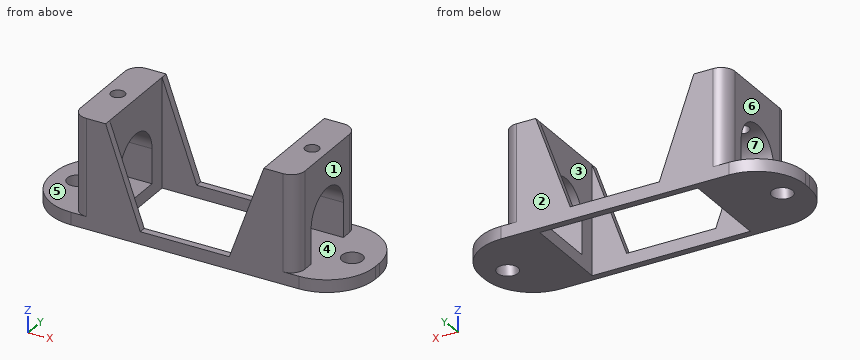
from build123d import *

# Parameters (mm, degrees)
F0_W      = 47
F0_H      = 15
F1_DEPTH  = 1.8
F3_DEPTH  = 14
F4_W      = 22.9
F4_H      = 13
F5_DEPTH  = 15.801
F6_R      = 1
F7_DEPTH  = 7
F8_R      = 1.5
F9_R      = 1.5
F10_DEPTH = 1.801
F12_DEPTH = 39.751
F13_R     = 7
F15_DEPTH = 1.001
F16_DEPTH = 14.001
F17_R     = 2


with BuildPart() as f1:
    # F0 (on Top) → F1 (new body)
    with BuildSketch(Plane.XY):
        with Locations((23.5, 7.5)):
            Rectangle(F0_W, F0_H)
    extrude(amount=F1_DEPTH)

    # F2 (on face) → F3 (join)
    with BuildSketch(Plane.XY.offset(1.8)):
        Polygon((39.75, 15), (23.5, 15), (7.25, 15), (7.25, 0), (23.5, 0), (39.75, 0), align=None)
    extrude(amount=F3_DEPTH)

    # F4 (on face) → F5 (cut, through all)
    with BuildSketch(Plane.XY.offset(15.8)):
        with Locations((23.5, 7.5)):
            Rectangle(F4_W, F4_H)
    extrude(amount=-F5_DEPTH, mode=Mode.SUBTRACT)

    # F6 (on face) → F7 (cut)
    with BuildSketch(Plane.XY.offset(15.8)):
        with Locations((9.45, 7.5)):
            Circle(F6_R)
        with Locations((37.55, 7.5)):
            Circle(F6_R)
    extrude(amount=-F7_DEPTH, mode=Mode.SUBTRACT)

    # F8 (on face) + F9 (on face) → F10 (cut, through all)
    with BuildSketch(Plane.XY.offset(1.8)):
        with Locations((3.625, 7.5)):
            Circle(F8_R)
    with BuildSketch(Plane.XY.offset(1.8)):
        with Locations((43.375, 7.5)):
            Circle(F9_R)
    extrude(amount=-F10_DEPTH, mode=Mode.SUBTRACT)

    # F11 (on face) → F12 (cut, through all)
    with BuildSketch(Plane(origin=(7.25, 0, 0), x_dir=(0, -1, 0), z_dir=(-1, 0, 0))):
        with BuildLine():
            Line((-11.5, 1.8), (-3.5, 1.8))
            Line((-3.5, 1.8), (-3.5, 6.8))
            ThreePointArc((-3.5, 6.8), (-7.5, 10.8), (-11.5, 6.8))
            Line((-11.5, 6.8), (-11.5, 1.8))
        make_face()
    extrude(amount=-F12_DEPTH, mode=Mode.SUBTRACT)

    # F13
    f13_edges = [f1.edges().sort_by_distance(p)[0] for p in [
        (0, 15, 0.9),
        (0, 0, 0.9),
        (47, 0, 0.9),
        (47, 15, 0.9),
    ]]
    fillet(f13_edges, radius=F13_R)

    # F14 (on face) → F15 (cut, through all)
    with BuildSketch(Plane.XZ.offset(-14)):
        Polygon((34.95, 15.8), (12.05, 15.8), (17.05, 1.8), (29.95, 1.8), align=None)
    extrude(amount=-F15_DEPTH, mode=Mode.SUBTRACT)

    # F14 (on face) → F16 (cut, through all)
    with BuildSketch(Plane.XZ.offset(-14)):
        Polygon((34.95, 15.8), (12.05, 15.8), (17.05, 1.8), (29.95, 1.8), align=None)
    extrude(amount=F16_DEPTH, mode=Mode.SUBTRACT)

    # F17
    f17_edges = [f1.edges().sort_by_distance(p)[0] for p in [
        (39.75, 15, 8.8),
        (39.75, 0, 8.8),
        (7.25, 0, 8.8),
        (7.25, 15, 8.8),
    ]]
    fillet(f17_edges, radius=F17_R)


solid = f1.part
Verification items for the finished model (mm, model axes). Face numbers are marked on the shaded views. A direction names the side the tool comes from. Give positions to 0.01 mm unless a question says otherwise; leave off trailing zeros. Order: outer loops, then holes, each group sorted by start corner. A loop starts at its lowest first (then second) coordinate and runs counter-clockwise, first axis right, second up. Notation, with made-up numbers: M 0,39.5 L 18,39.5 A20 ccw 18,60.5 Z; hole C 86,13.5 d11. An arc over 180 degrees is marked long. Answer as a JSON object with one key per item and string values. Group by question number.
1) Cross-section at B-B (x = 34.5). Enter the section's corners in (y, z).
2) Depth check by flat-ended pin: pin 1 Ø1.5 at (y, z) = (6, 12) entering from +X; pin 2 Ø3.5 at (y, z) = (7.5, 8.5) entering from -X; pin 3 Ø3.5 at (x, y) = (3.625, 7.5) entering from +Z. Enter the tip coordinate at first touch or a pass-through.
3) Cross-section at C-C (x = 10). Enter the section's corners in (y, z), then the cut area to 3 significant figures.
4) Cross-section at A-A (z = 2.5). Enter the section's corners in (x, y).
5) Access from +Z, -Z, +X, -X, +Y, -Y to the whole of each face (thin tool, end or side, straight path). Record for the marked faces 4, 5, 6 and 7.
6) Cross-section at D-D (z = 5.5). Enter the section's corners in (x, y), then the cut area to 3 significant figures.
7) Mould release check, pull along Y, two halves, no side actions. Record for the marked faces 1, 2 and 3: released by +Y, released by -Y, zero draft, split by the parting line, or undercut.
8) Scan lines: line 1 along X through (y, z) = (7.5, 14.4); line 2 along Y through (x, z) = (37.55, 12.45); line 3 along Y through (x, z) = (33, 1). Record each from-to range of solid material in increasing order. Write a range as [from, to].
Result sheet:
{
 "1": {"outline": "M 0,0 L 1,0 L 1,14.54 L 0,14.54 Z; M 14,0 L 15,0 L 15,14.54 L 14,14.54 Z"},
 "2": {"pin 1": "stops at x = 39.75", "pin 2": "passes through", "pin 3": "stops at z = 1.8"},
 "3": {"outline": "M 0,0 L 15,0 L 15,15.8 L 8.34,15.8 L 8.34,10.71 A4 cw 11.5,6.8 L 11.5,1.8 L 3.5,1.8 L 3.5,6.8 A4 cw 6.66,10.71 L 6.66,15.8 L 0,15.8 Z", "area": "163 mm2"},
 "4": {"outline": "M 7.25,2 A2 ccw 9.25,0 L 16.8,0 L 16.8,1 L 12.05,1 L 12.05,3.5 L 7.25,3.5 Z; M 7.25,11.5 L 12.05,11.5 L 12.05,14 L 16.8,14 L 16.8,15 L 9.25,15 A2 ccw 7.25,13 Z; M 30.2,0 L 37.75,0 A2 ccw 39.75,2 L 39.75,3.5 L 34.95,3.5 L 34.95,1 L 30.2,1 Z; M 30.2,14 L 34.95,14 L 34.95,11.5 L 39.75,11.5 L 39.75,13 A2 ccw 37.75,15 L 30.2,15 Z"},
 "5": {"face 4": "+X", "face 5": "-X", "face 6": "+Z, -X, +Y, -Y", "face 7": "+X, -X"},
 "6": {"outline": "M 7.25,2 A2 ccw 9.25,0 L 15.73,0 L 15.73,1 L 12.05,1 L 12.05,3.5 L 7.25,3.5 Z; M 7.25,11.5 L 12.05,11.5 L 12.05,14 L 15.73,14 L 15.73,15 L 9.25,15 A2 ccw 7.25,13 Z; M 31.27,0 L 37.75,0 A2 ccw 39.75,2 L 39.75,3.5 L 34.95,3.5 L 34.95,1 L 31.27,1 Z; M 31.27,14 L 34.95,14 L 34.95,11.5 L 39.75,11.5 L 39.75,13 A2 ccw 37.75,15 L 31.27,15 Z", "area": "78.5 mm2"},
 "7": {"face 1": "zero draft", "face 2": "released by +Y", "face 3": "undercut"},
 "8": {"line 1": "x = [7.25, 8.45], [10.45, 12.05], [34.95, 36.55], [38.55, 39.75]", "line 2": "y = [0, 6.5], [8.5, 15]", "line 3": "y = [0, 1], [14, 15]"}
}
